from build123d import *

# Parameters (mm, degrees)
SKETCH2_W             = 5
SKETCH2_H             = 10
BOSS_EXTRUDE1_DEPTH   = 48
SKETCH2_W_2           = 10
SKETCH2_H_2           = 5
BOSS_EXTRUDE1_2_DEPTH = 48
BOSS_EXTRUDE1_3_DEPTH = 48
BOSS_EXTRUDE1_4_DEPTH = 48
SKETCH3_W             = 165
SKETCH3_H             = 55.28
BOSS_EXTRUDE2_DEPTH   = 3
SKETCH4_W             = 10
SKETCH4_H             = 3.86
BOSS_EXTRUDE3_DEPTH   = 3
SKETCH5_W             = 10
SKETCH5_H             = 5
BOSS_EXTRUDE4_DEPTH   = 10
SKETCH7_W             = 5
SKETCH7_H             = 10
BOSS_EXTRUDE5_DEPTH   = 10
SKETCH8_R             = 1.73
CUT_EXTRUDE1_DEPTH    = 6
SKETCH10_W            = 10
SKETCH10_H            = 8.5
SKETCH10_W_2          = 1.85
SKETCH10_H_2          = 10
BOSS_EXTRUDE6_DEPTH   = 3
SKETCH11_R            = 1.75
CUT_EXTRUDE3_DEPTH    = 52
SKETCH12_W            = 82.72
SKETCH12_H            = 54.46
SKETCH12_W_2          = 81.92
SKETCH12_H_2          = 53.66
CUT_EXTRUDE4_DEPTH    = 0.28
CUT_EXTRUDE5_DEPTH    = 4


with BuildPart() as part:
    # Sketch2 → Boss-Extrude1 (new body)
    with BuildSketch(Plane.XY):
        with Locations((-74.585, 0)):
            Rectangle(SKETCH2_W, SKETCH2_H)
    extrude(amount=BOSS_EXTRUDE1_DEPTH)



with BuildPart() as body_2:
    # Sketch2 → Boss-Extrude1 2 (new body)
    with BuildSketch(Plane.XY):
        with Locations((0, 29)):
            Rectangle(SKETCH2_W_2, SKETCH2_H_2)
    extrude(amount=BOSS_EXTRUDE1_2_DEPTH)


with BuildPart() as body_3:
    # Sketch2 → Boss-Extrude1 3 (new body)
    with BuildSketch(Plane.XY):
        with Locations((74.585, 0)):
            Rectangle(SKETCH2_W, SKETCH2_H)
    extrude(amount=BOSS_EXTRUDE1_3_DEPTH)


with BuildPart() as body_4:
    # Sketch2 → Boss-Extrude1 4 (new body)
    with BuildSketch(Plane.XY):
        with Locations((0, -29)):
            Rectangle(SKETCH2_W_2, SKETCH2_H_2)
    extrude(amount=BOSS_EXTRUDE1_4_DEPTH)


with BuildPart() as part_1:
    add(part.part)

    add(body_2.part)  # Boss-Extrude2 merges body 2

    add(body_3.part)  # Boss-Extrude2 merges body 3

    add(body_4.part)  # Boss-Extrude2 merges body 4
    # Sketch3 → Boss-Extrude2 (add)
    with BuildSketch(Plane.XY.offset(48)):
        Rectangle(SKETCH3_W, SKETCH3_H)
    extrude(amount=BOSS_EXTRUDE2_DEPTH)

    # Sketch4 → Boss-Extrude3 (add)
    with BuildSketch(Plane.XY.offset(48)):
        with Locations((0, 29.57)):
            Rectangle(SKETCH4_W, SKETCH4_H)
        with Locations((0, -29.57)):
            Rectangle(SKETCH4_W, SKETCH4_H)
    extrude(amount=BOSS_EXTRUDE3_DEPTH)

    # Sketch5 → Boss-Extrude4 (add)
    with BuildSketch(Plane(origin=(0, 5, 0), x_dir=(1, 0, 0), z_dir=(0, 1, 0))):
        with Locations((-82.085, -2.5)):
            Rectangle(SKETCH5_W, SKETCH5_H)
        with Locations((82.085, -2.5)):
            Rectangle(SKETCH5_W, SKETCH5_H)
    extrude(amount=-BOSS_EXTRUDE4_DEPTH)

    # Sketch7 → Boss-Extrude5 (add)
    with BuildSketch(Plane.ZY.offset(5)):
        with Locations((2.5, 36.5)):
            Rectangle(SKETCH7_W, SKETCH7_H)
        with Locations((2.5, -36.5)):
            Rectangle(SKETCH7_W, SKETCH7_H)
    extrude(amount=-BOSS_EXTRUDE5_DEPTH)

    # Sketch8 → Cut-Extrude1 (cut, through all)
    with BuildSketch(Plane.XY.offset(5)):
        with Locations((-82.085, 0)):
            Circle(SKETCH8_R)
        with Locations((0, -36.5)):
            Circle(SKETCH8_R)
        with Locations((82.085, 0)):
            Circle(SKETCH8_R)
        with Locations((0, 36.5)):
            Circle(SKETCH8_R)
    extrude(amount=-CUT_EXTRUDE1_DEPTH, mode=Mode.SUBTRACT)

    # Sketch10 → Boss-Extrude6 (add)
    with BuildSketch(Plane.XY.offset(51)):
        with Locations((32.52, 31.89)):
            Rectangle(SKETCH10_W, SKETCH10_H)
        with Locations((69.005, -20.32)):
            Rectangle(SKETCH10_W_2, SKETCH10_H_2)
    extrude(amount=-BOSS_EXTRUDE6_DEPTH)

    # Sketch11 → Cut-Extrude3 (cut, through all)
    with BuildSketch(Plane.XY.offset(51)):
        with Locations((32.52, 31.75)):
            Circle(SKETCH11_R)
        with Locations((65.54, -20.32)):
            Circle(SKETCH11_R)
    extrude(amount=-CUT_EXTRUDE3_DEPTH, mode=Mode.SUBTRACT)

    # Sketch12 → Cut-Extrude4 (cut)
    with BuildSketch(Plane.XY.offset(51)):
        with Locations((-30.625, 0)):
            Rectangle(SKETCH12_W, SKETCH12_H)
        with Locations((-30.625, 0)):
            Rectangle(SKETCH12_W_2, SKETCH12_H_2, mode=Mode.SUBTRACT)
    extrude(amount=-CUT_EXTRUDE4_DEPTH, mode=Mode.SUBTRACT)

    # Sketch13 → Cut-Extrude5 (cut, through all)
    with BuildSketch(Plane(origin=(0, 0, 48), x_dir=(-1, 0, 0), z_dir=(0, 0, -1))):
        Polygon((82.5, -27.64), (82.5, 27.64), (72.085, 27.64), (72.085, 5), (77.085, 5), (77.085, -5), (72.085, -5), (72.085, -27.64), align=None)
        Polygon((-82.5, 27.64), (-82.5, -27.64), (-72.085, -27.64), (-72.085, -5), (-77.085, -5), (-77.085, 5), (-72.085, 5), (-72.085, 27.64), align=None)
    extrude(amount=-CUT_EXTRUDE5_DEPTH, mode=Mode.SUBTRACT)


solid = part_1.part
Design review of the part built by this model. Coordinates are the model's own, in mm. A direction names the side the tool comes from. Coordinates: 2 decimals unless noted, no trailing zeros. Loops run counter-clockwise (first coordinate to the right, second up) from the corner with the lowest first, then second, coordinate; pieces in that order, holes last. Notation, with made-up numbers: (0.25, 0.25) -> (15.25, 0.25) arc R6 cw to (15.25, 5.25) -> close; hole circle Ø9 at (68, 59). An arc over 180 degrees is marked (long way). Use a Markdown table: item, result. Add a question column.
Item 1: We need section C-C, the plane x = 0. Write out the cut boundary in (y, z), and give its area (3 significant figures).
Item 2: We need section B-B, the plane z = 37.5. Write out the cut boundary in (x, y) (3 decimals), and give its area (3 significant figures).
Item 3: Machinability: for faces 4 (the flat face through (-72.085, 0, 24)), 5 (the flat face through (38, -27.64, 49)), 6 (the flat face through (37.52, 32, 50)), 7 (the flat face through (0, -26.5, 24)), which of the approach directions +Z, -Z, +X, -X, +Y, -Y give a long, thin tool a straight path to every point of the face, cutting with its end or side? Answer none if there is none.
Item 4: Wall thickness on L1, parallel to Y at x = 0, z = 2.1; L2, parallel to X at y = -1.5, z = 44 (3 decimals); L3, parallel to Z at x = 65, y = 5: over which ranges is each line inside the solid? List them lowest first. Write a range as from..to.
Item 5: We need section D-D, the plane y = -36.5. Write out the cut boundary in (x, z).
Item 6: The part is to be moulded in two halves that separate along X. For faces 1 (the flat face through (77.085, 0, 28)), 2 (the cylindrical face through (-83.813, 0.076, 2.535)), 3 (the flat face through (-84, 0, 5)), say which applies: +X half, -X half, draft (parallel to the pull), parting line (faces both ways), or undercut.
Item 7: We need section A-A, the plane y = 0. Write out the cut boundary in (x, z) (3 decimals), and give its area (3 significant figures).
Item 8: Clearance check with flat-ended pins moving along their axes: P1, Ø1.5, axis at y = -21, z = 49, coming from the +X side (3 decimals); P2, Ø3, axis at y = -31.5, z = 36, coming from the -X side; P3, Ø5, axis at y = -1.5, z = 20, coming from the -X side (3 decimals); P4, Ø11, axis at x = -1, y = -36.5, coming from the +Z side. State where each tip first meets the part, or that it passes through.
Numbers:
| question | item | result |
|---|---|---|
| 1 | outline | (-41.5, 0) -> (-38.23, 0) -> (-38.23, 5) -> (-41.5, 5) -> close; (-34.77, 0) -> (-26.5, 0) -> (-26.5, 48) -> (26.5, 48) -> (26.5, 0) -> (34.77, 0) -> (34.77, 5) -> (31.5, 5) -> (31.5, 51) -> (27.23, 51) -> (27.23, 50.72) -> (26.83, 50.72) -> (26.83, 51) -> (-26.83, 51) -> (-26.83, 50.72) -> (-27.23, 50.72) -> (-27.23, 51) -> (-31.5, 51) -> (-31.5, 5) -> (-34.77, 5) -> close; (38.23, 0) -> (41.5, 0) -> (41.5, 5) -> (38.23, 5) -> close |
| 1 | area | 734 mm^2 |
| 2 | outline | (-77.085, -5) -> (-72.085, -5) -> (-72.085, 5) -> (-77.085, 5) -> close; (-5, -31.5) -> (5, -31.5) -> (5, -26.5) -> (-5, -26.5) -> close; (-5, 26.5) -> (5, 26.5) -> (5, 31.5) -> (-5, 31.5) -> close; (72.085, -5) -> (77.085, -5) -> (77.085, 5) -> (72.085, 5) -> close |
| 2 | area | 200 mm^2 |
| 3 | face 4 | -Z, +Y, -Y |
| 3 | face 5 | +Z, -Z, +X, -Y |
| 3 | face 6 | +Z, -Z, +X, +Y |
| 3 | face 7 | -Z, +X, -X |
| 4 | L1 | y = -41.5..-38.23, -34.77..-26.5, 26.5..34.77, 38.23..41.5 |
| 4 | L2 | x = -77.085..-72.085, 72.085..77.085 |
| 4 | L3 | z = 48..51 |
| 5 | outline | (-5, 0) -> (-1.73, 0) -> (-1.73, 5) -> (-5, 5) -> close; (1.73, 0) -> (5, 0) -> (5, 5) -> (1.73, 5) -> close |
| 6 | face 1 | +X half |
| 6 | face 2 | undercut |
| 6 | face 3 | draft |
| 7 | outline | (-87.085, 0) -> (-83.815, 0) -> (-83.815, 5) -> (-87.085, 5) -> close; (-80.355, 0) -> (-72.085, 0) -> (-72.085, 48) -> (72.085, 48) -> (72.085, 0) -> (80.355, 0) -> (80.355, 5) -> (77.085, 5) -> (77.085, 51) -> (10.735, 51) -> (10.735, 50.72) -> (10.335, 50.72) -> (10.335, 51) -> (-71.585, 51) -> (-71.585, 50.72) -> (-71.985, 50.72) -> (-71.985, 51) -> (-77.085, 51) -> (-77.085, 5) -> (-80.355, 5) -> close; (83.815, 0) -> (87.085, 0) -> (87.085, 5) -> (83.815, 5) -> close |
| 7 | area | 1,010 mm^2 |
| 8 | P1 | stops at x = 72.085 |
| 8 | P2 | stops at x = -5 |
| 8 | P3 | stops at x = -77.085 |
| 8 | P4 | stops at z = 51 |
